Study the drawing (mm; zero at the part's minimum x, y, z) and answer. Give positions to 0.01 mm unless a question says otherwise; leave off trailing zeros. Loops run counter-clockwise (first coordinate to the right, second up) from the corner with the lowest first, then second, coordinate; pieces in that order, holes last. Notation, with made-up numbers: M -36,2.25 L 0,2.25 A27 ccw 0,28.25 Z; hole C 40,58 d5. An arc over 180 degrees is marked long. Return JSON: item names as keys, results as strings.
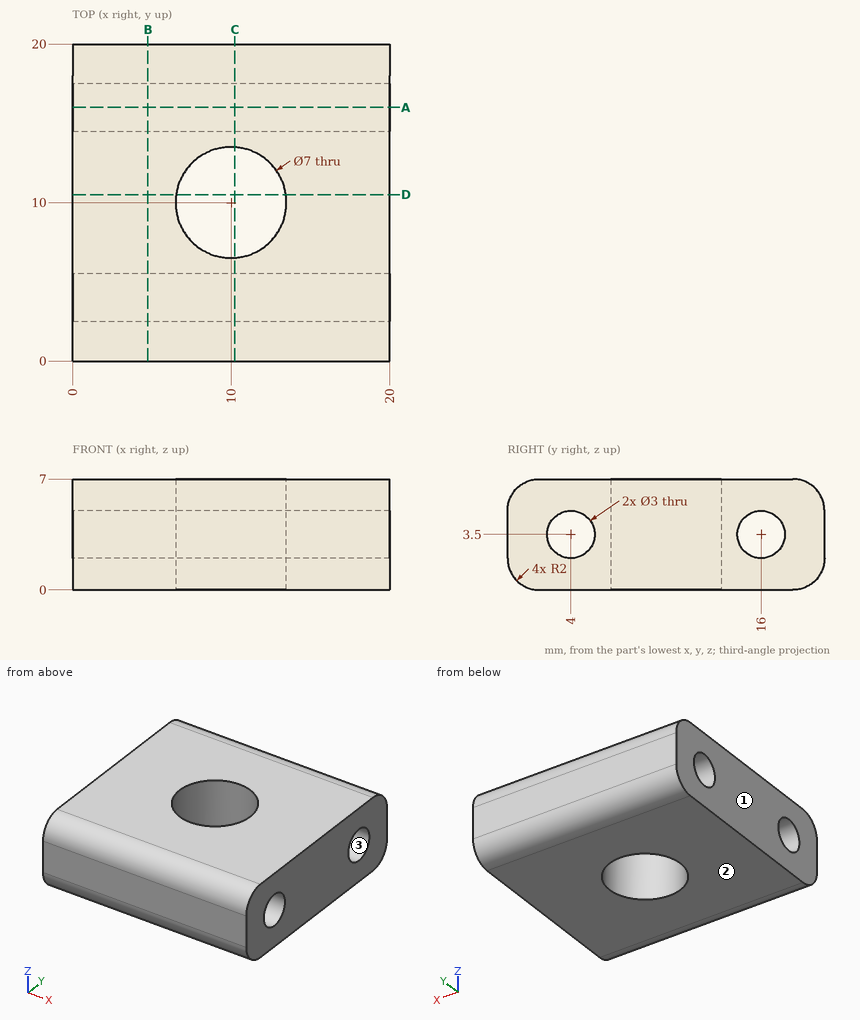
(1) Given pin 1 (2 mm diameter, centred on y = 14, z = 5.5, fed in from -X), flat-ended and moving along its own axis, determine where the tip first touches the part or whether it passes through.
Values follow:
{"pin 1": "x = 0"}
(2) The part is cut by section D-D (y = 10.5). Determine the outline of the cut face in (x, z).
Values follow:
{"outline": "M 0,0 L 6.54,0 L 6.54,7 L 0,7 Z; M 13.46,0 L 20,0 L 20,7 L 13.46,7 Z"}
(3) Straight lines are drawn through the part: line 1 along Y through (x, z) = (8.25, 2.25); line 2 along Y through (x, z) = (3, 3.25); line 3 along Z through (x, y) = (12.5, 16). For each, find the intervals that lie inside material, in ascending order.
Values follow:
{"line 1": "0 to 3.17, 4.83 to 6.97, 13.03 to 15.17, 16.83 to 20", "line 2": "0 to 2.52, 5.48 to 14.52, 17.48 to 20", "line 3": "0 to 2, 5 to 7"}
(4) The part is cut by section C-C (x = 10.25). Determine the outline of the cut face in (y, z).
Values follow:
{"outline": "M 0,2 A2 ccw 2,0 L 6.51,0 L 6.51,7 L 2,7 A2 ccw 0,5 Z; M 13.49,0 L 18,0 A2 ccw 20,2 L 20,5 A2 ccw 18,7 L 13.49,7 Z; hole C 4,3.5 d3; hole C 16,3.5 d3"}
(5) Determine the mould class of the marked faces 1, 2 and 3 for opening direction Z: released by +Z, released by -Z, zero draft, split by the parting line, or undercut.
Values follow:
{"face 1": "zero draft", "face 2": "released by -Z", "face 3": "undercut"}
(6) The part is cut by section A-A (y = 16). Determine the outline of the cut face in (x, z).
Values follow:
{"outline": "M 0,0 L 20,0 L 20,2 L 0,2 Z; M 0,5 L 20,5 L 20,7 L 0,7 Z"}
(7) The part is cut by section B-B (x = 4.75). Determine the outline of the cut face in (y, z), and give its area (3 significant figures).
Values follow:
{"outline": "M 0,2 A2 ccw 2,0 L 18,0 A2 ccw 20,2 L 20,5 A2 ccw 18,7 L 2,7 A2 ccw 0,5 Z; hole C 4,3.5 d3; hole C 16,3.5 d3", "area": "122 mm²"}
